```python
from build123d import *

# Parameters (mm, degrees)
F0_R            = 38.1
F0_R_2          = 19.05
F1_DEPTH        = 63.5
F3_COPIES_COUNT = 4
F4_R            = 109.5375
F5_DEPTH        = 38.101
F5_DEPTH_BACK   = 38.101


# Not quite as in the source:
# - a pattern or mirror of a feature is missing from the dataset's text; its kind, count and spacing are read off the source's solid


with BuildPart() as f1:
    # F0 (on Top) → F1 (new body)
    with BuildSketch(Plane.XY):
        Circle(F0_R)
        Circle(F0_R_2, mode=Mode.SUBTRACT)
    extrude(amount=F1_DEPTH)

    # F2 (on Front) → F3 (revolve, cut)
    with BuildSketch(Plane.XZ):
        Polygon((28.575, 0), (28.575, 63.5), (23.8125, 63.5), (23.8125, 58.674), (25.7683, 58.674), (25.7683, 0), align=None)
    f3 = revolve(axis=Axis((28.575, 0, 28.6447224574), (0, 0, -1)), mode=Mode.SUBTRACT)

    # F3_copies: F3 ×4 about axis
    f3_copies_axis = Axis((0, 0, 0), (0, 0, 1))
    for i in range(1, F3_COPIES_COUNT):
        add(f3.rotate(f3_copies_axis, i * 360 / F3_COPIES_COUNT), mode=Mode.SUBTRACT)

    # F4 (on Front) → F5 (cut, two sides)
    with BuildSketch(Plane.XZ) as f5_sk:
        with Locations((0, -101.6)):
            Circle(F4_R)
    extrude(amount=-F5_DEPTH, mode=Mode.SUBTRACT)
    extrude(f5_sk.sketch, amount=F5_DEPTH_BACK, mode=Mode.SUBTRACT)


solid = f1.part
```
Verification items for the finished model (mm, model axes). A direction names the side the tool comes from. Give positions to 0.01 mm unless a question says otherwise; leave off trailing zeros. Loops run counter-clockwise (first coordinate to the right, second up) from the corner with the lowest first, then second, coordinate; pieces in that order, holes last.
1. Section check A-A, the plane x = 0. Enter the section's corners in (y, z).
2. Section check D-D, the plane x = -9. Enter the section's corners in (y, z), then the cut area to 3 significant figures.
3. Section check C-C, the plane z = 26.5. Enter the section's corners in (x, y) (3 decimals), then the cut area to 3 significant figures.
4. Thickness scan on line 1 (X direction, y = 7, z = 33); line 2 (X direction, y = 16.5, z = 47); line 3 (Z direction, x = 19, y = 12). Record the ranges inside material, lowest first.
5. Set-up check for faces 1 (the cylindrical face through (32.354, -2.898, 61.053)), 2 (the cylindrical face through (-25.898, -0.843, 30.622)): record each of +Z, -Z, +X, -X, +Y, -Y from which the full face is reachable in a straight line by a thin tool's end or side.
6. Go/stop test with flat-tipped pins: pin 1 Ø4 at (x, z) = (30.5, 22.5) entering from -Y; pin 2 Ø5.5 at (x, y) = (28.575, 0) entering from +Z; pin 3 Ø8.5 at (x, y) = (0, -28.575) entering from -Z (3 decimals); pin 4 Ø12 at (x, z) = (-12, 18) entering from +Y. Record where each tip stops, or that it passes through.
7. Mould release check, pull along Y, two halves, no side actions. Record for faces 3 (the cylindrical face through (-2.898, -32.354, 61.053)), 4 (the cylindrical face through (-8.259, -37.194, 31.862)), 5 (the flat face through (7.9, 17.5, 63.5)): released by +Y, released by -Y, zero draft, split by the parting line, or undercut.
8. Section check B-B, the plane y = 0. Count the separate pieces of the cut face and the enclosed holes in it, then the cut area to 3 significant figures.
Geometry says:
1. outline: (-38.1, 7.94) - (-31.38, 7.94) - (-31.38, 58.67) - (-33.34, 58.67) - (-33.34, 63.5) - (-38.1, 63.5) - close; (-25.77, 7.94) - (-19.05, 7.94) - (-19.05, 63.5) - (-23.81, 63.5) - (-23.81, 58.67) - (-25.77, 58.67) - close; (19.05, 7.94) - (25.77, 7.94) - (25.77, 58.67) - (23.81, 58.67) - (23.81, 63.5) - (19.05, 63.5) - close; (31.38, 7.94) - (38.1, 7.94) - (38.1, 63.5) - (33.34, 63.5) - (33.34, 58.67) - (31.38, 58.67) - close
2. outline: (-37.02, 7.57) - (-16.79, 7.57) - (-16.79, 63.5) - (-37.02, 63.5) - close; (16.79, 7.57) - (37.02, 7.57) - (37.02, 63.5) - (16.79, 63.5) - close
2. area: 2,260 mm2
3. outline: circle Ø76.2 at (0, 0); hole circle Ø5.613 at (-28.575, 0); hole circle Ø38.1 at (0, 0); hole circle Ø5.613 at (0, -28.575); hole circle Ø5.613 at (0, 28.575); hole circle Ø5.613 at (28.575, 0)
3. area: 3,320 mm2
4. line 1: x = -37.45 to -17.72, 17.72 to 37.45
4. line 2: x = -34.34 to -9.52, 9.52 to 34.34
4. line 3: z = 6.28 to 63.5
5. face 1: +Z
5. face 2: +Z, -Z
6. pin 1: stops at y = -25.29
6. pin 2: passes through
6. pin 3: stops at z = 7.855
6. pin 4: stops at y = 37.62
7. face 3: undercut
7. face 4: split by the parting line
7. face 5: zero draft
8. separate pieces: 4
8. enclosed holes: 0
8. area: 1,560 mm2
